Design review of the part shown in the three views and the two pictorial views. Dimensions are in mm from the part's minimum x, y and z. Give positions to 0.01 mm unless a question says otherwise; leave off trailing zeros. Order: outer loops, then holes, each group sorted by start corner. A loop starts at its lowest first (then second) coordinate and runs counter-clockwise, first axis right, second up.
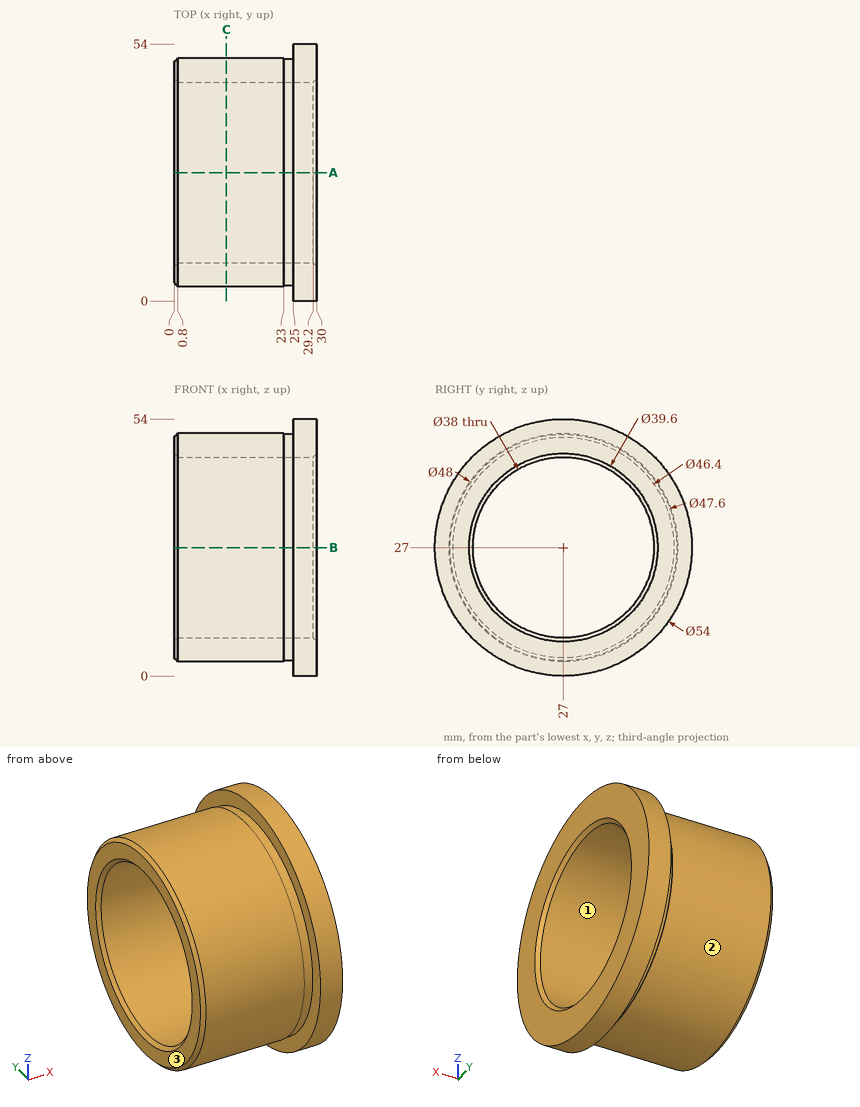
Item 1: Clearance check with flat-ended pins moving along their axes: pin 1 Ø3 at (x, y) = (6, 23) entering from -Z; pin 2 Ø5 at (x, z) = (7, 20.5) entering from -Y; pin 3 Ø3 at (x, y) = (4, 35.5) entering from +Z. State where each tip first meets the part, or that it passes through.
Values found:
pin 1: stops at z = 3.13
pin 2: stops at y = 3.34
pin 3: stops at z = 49.96
Item 2: For line 1 (Y direction, x = 9, z = 27); line 2 (Y direction, x = 19.5, z = 16); line 3 (Z direction, x = 14, y = 17.5), list the stretches that pass through material, from the lowest coordinate up.
Values found:
line 1: y = 3 to 8, 46 to 51
line 2: y = 5.67 to 11.51, 42.49 to 48.33
line 3: z = 4.96 to 10.55, 43.45 to 49.04
Item 3: Take a section at C-C (x = 11). Give the boundary of the cut face in (y, z), and give its area (3 significant figures).
Values found:
outline: circle Ø48 at (27, 27); hole circle Ø38 at (27, 27)
area: 675 mm2
Item 4: Take a section at A-A (y = 27). Give the boundary of the cut face in (x, z).
Values found:
outline: (0, 3.8) - (0.8, 3) - (23, 3) - (23, 3.2) - (25, 3.2) - (25, 0) - (30, 0) - (30, 7.2) - (29.2, 8) - (0.8, 8) - (0, 7.2) - close; (0, 46.8) - (0.8, 46) - (29.2, 46) - (30, 46.8) - (30, 54) - (25, 54) - (25, 50.8) - (23, 50.8) - (23, 51) - (0.8, 51) - (0, 50.2) - close
Item 5: Draft analysis for pull direction Z (two halves, no side actions). For the marked faces 1, 2 and 3, state which applies: released by +Z, released by -Z, zero draft, split by the parting line, or undercut.
Values found:
face 1: undercut
face 2: split by the parting line
face 3: zero draft
